```python
from build123d import *

# Parameters (mm, degrees)
SKETCH1_R                       = 3
SKETCH1_R_2                     = 6
BOSS_EXTRUDE1_DEPTH             = 6
M4X0_7_TAPPED_HOLE1_D           = 3.3
CHAMFER1_SIZE                   = 3
CHAMFER2_SIZE                   = 1
BOSS_EXTRUDE2_DEPTH             = 4.25
M4X0_7_START                    = -20.526744186
M4X0_7_TAPPED_HOLE3_OUTLINE_R   = 1.65
M4X0_7_TAPPED_HOLE3_DEPTH       = 1.123131525
M4X0_7_START_2                  = -19.403612661
M4X0_7_TAPPED_HOLE3_2_OUTLINE_R = 1.65
M4X0_7_TAPPED_HOLE3_2_DEPTH     = 0.494491736
M4X0_7_START_3                  = -6.0000001
M4X0_7_TAPPED_HOLE3_3_DEPTH     = 6.0000002
M4X0_7_START_4                  = -6.7750001
M4X0_7_TAPPED_HOLE3_4_DEPTH     = 0.775
SKETCH14_R                      = 3
CUT_EXTRUDE1_DEPTH              = 87.67199356


with BuildPart() as part:
    # Sketch1 → Boss-Extrude1 (new body)
    with BuildSketch(Plane.XY):
        with BuildLine():
            Line((62.473255814, 56.275636954), (55.545052584, 60.275636954))
            Line((55.545052584, 60.275636954), (24.782656891, 6.993604651))
            ThreePointArc((24.782656891, 6.993604651), (21.122402853, 3.333350613), (16.122402853, 1.993604651))
            Line((16.122402853, 1.993604651), (-20.526744186, 1.993604651))
            Line((-20.526744186, 1.993604651), (-20.526744186, -13.006395349))
            Line((-20.526744186, -13.006395349), (22.473255814, -13.006395349))
            Line((22.473255814, -13.006395349), (62.473255814, 56.275636954))
        make_face()
        with Locations((-16.403612561, -5.506395349)):
            Circle(SKETCH1_R, mode=Mode.SUBTRACT)
        with Locations((17.535345593, -5.506395349)):
            Circle(SKETCH1_R_2, mode=Mode.SUBTRACT)
    extrude(amount=-BOSS_EXTRUDE1_DEPTH)

    # M4x0.7 Tapped Hole1 (through all)
    with Locations(Plane.XY):
        with Locations((36.509154199, 19.304493784)):
            Hole(M4X0_7_TAPPED_HOLE1_D / 2)

    # Chamfer1
    chamfer1_edges = [part.edges().sort_by_distance(p)[0] for p in [
        (-20.526744186, -13.006395349, -3),
    ]]
    chamfer(chamfer1_edges, length=CHAMFER1_SIZE)

    # Chamfer2
    chamfer2_edges = [part.edges().sort_by_distance(p)[0] for p in [
        (42.473255814, 21.634620803, -6),
        (55.545052584, 60.275636954, -3),
        (42.473255814, 21.634620803, 0),
    ]]
    chamfer(chamfer2_edges, length=CHAMFER2_SIZE)

    # Sketch6 → Boss-Extrude2 (add)
    with BuildSketch(Plane(origin=(0, 0, -6), x_dir=(-1, 0, 0), z_dir=(0, 0, -1))):
        Polygon((20.526744186, 1.993604651), (1.306644629, 1.993604651), (1.306644629, -13.006395349), (17.526744186, -13.006395349), (20.526744186, -10.006395349), align=None)
    extrude(amount=BOSS_EXTRUDE2_DEPTH)

    # M4x0.7 Tapped Hole3: read off the stored shape, not the designer's step
    # M4x0.7 Tapped Hole3 outline → M4x0.7 Tapped Hole3 (cut)
    with BuildSketch(Plane.YZ.offset(M4X0_7_START)):
        with Locations((-5.506395349, -5.125)):
            Circle(M4X0_7_TAPPED_HOLE3_OUTLINE_R)
    extrude(amount=M4X0_7_TAPPED_HOLE3_DEPTH, mode=Mode.SUBTRACT)

    # M4x0.7 Tapped Hole3 2 outline → M4x0.7 Tapped Hole3 2 (cut)
    with BuildSketch(Plane.YZ.offset(M4X0_7_START_2)):
        with Locations((-5.506395349, -5.125)):
            Circle(M4X0_7_TAPPED_HOLE3_2_OUTLINE_R)
    extrude(amount=M4X0_7_TAPPED_HOLE3_2_DEPTH, mode=Mode.SUBTRACT)

    # M4x0.7 Tapped Hole3 3 outline → M4x0.7 Tapped Hole3 3 (cut)
    with BuildSketch(Plane.XY.offset(M4X0_7_START_3)):
        with BuildLine():
            ThreePointArc((-18.909118414, -3.856413403), (-18.986363136, -3.980158321), (-19.057501217, -4.107511865))
            ThreePointArc((-19.057501217, -4.107511865), (-19.403612561, -5.506395898), (-19.057500704, -6.905279805))
            ThreePointArc((-19.057500704, -6.905279805), (-18.98636247, -7.032633505), (-18.909117577, -7.156378566))
            Line((-18.909117577, -7.156378566), (-18.909118414, -3.856413403))
        make_face()
    extrude(amount=M4X0_7_TAPPED_HOLE3_3_DEPTH, mode=Mode.SUBTRACT)

    # M4x0.7 Tapped Hole3 4 outline → M4x0.7 Tapped Hole3 4 (add)
    with BuildSketch(Plane.XY.offset(M4X0_7_START_4)):
        with BuildLine():
            ThreePointArc((-18.909118414, -3.856413403), (-18.986363136, -3.980158321), (-19.057501217, -4.107511865))
            ThreePointArc((-19.057501217, -4.107511865), (-19.403612561, -5.506395898), (-19.057500704, -6.905279805))
            ThreePointArc((-19.057500704, -6.905279805), (-18.98636247, -7.032633505), (-18.909117577, -7.156378566))
            Line((-18.909117577, -7.156378566), (-18.909118414, -3.856413403))
        make_face()
    extrude(amount=M4X0_7_TAPPED_HOLE3_4_DEPTH)

    # Sketch14 → Cut-Extrude1 (cut, through all)
    with BuildSketch(Plane.XY.offset(-6)):
        with Locations((-16.403612561, -5.506395349)):
            Circle(SKETCH14_R)
    extrude(amount=-CUT_EXTRUDE1_DEPTH, mode=Mode.SUBTRACT)


solid = part.part
```
Geometry: final body of the model. Coordinates: model frame, mm. A direction names the side the tool comes from. Round coordinates to 2 decimals unless told otherwise and drop trailing zeros. Order: outer loops, then holes, each group sorted by start corner. A loop starts at its lowest first (then second) coordinate and runs counter-clockwise, first axis right, second up. Notation, with made-up numbers: (3, -27) -> (42, -27) arc R12 ccw to (42, -15) -> close; hole circle Ø2 at (10, -30.5). An arc over 180 degrees is marked (long way). Use CSV: the item, a comma, the result in double quotes. Start each with the question number.
1) Material intervals for line 1 along X through (y, z) = (-3.5, -0.5); line 2 along Y through (x, z) = (-0.5, -3); line 3 along Z through (x, y) = (29.5, 8.5), sorted ascending. Write a range as from..to.
2) Section A-A (z = -8). Return the cut outline in (x, y), and give its area (3 significant figures).
3) Section C-C (y = 46.5). Return the cut outline in (x, z), and give its area (3 significant figures).
4) Draft query along X for faces 6 (the face through (-19.006, -11.527, -5.053)), 7 (the face through (35.622, 20.696, -3.042)), 8 (the face through (59.485, 58.001, -2.958)). Return one class per face: +X half, -X half, draft (parallel to the pull), parting line (faces both ways), or undercut.
5) First-contact query: pin 1 Ø4.5 at (y, z) = (-4.5, -8.5) entering from +X; pin 2 Ø4.5 at (x, y) = (36.51, 19.3) entering from +Z; pin 3 Ø2.5 at (y, z) = (-5.51, -5.12) entering from -X; pin 4 Ø4 at (y, z) = (1, -1.5) entering from +X. Flat tips, straight axial feed; report the tip coordinate or a pass-through.
6) Section B-B (x = 0). Return the cut outline in (y, z).
7) Set-up query: faces 1 (the face through (41.608, 21.15, -5.507)), 2 (the face through (-7, 1.994, -4)), 3 (the face through (-19.9, -4, -5.8)), 4 (the face through (30, 15, -6)), 5 (the face through (-13.54, -4.61, -5.05)). Return all of +Z, -Z, +X, -X, +Y, -Y with unobstructed straight access to the full face (end or side cutting, diameter ignored); none if empty.
8) Section D-D (x = -11.5). Return the cut outline in (y, z), and give its area (3 significant figures).
Returned:
1,line 1,"x = -20.53..-18.63, -14.17..11.88, 23.19..27.38"
1,line 2,"y = -13.01..1.99"
1,line 3,"z = -6..0"
2,outline,"(-20.53, -10.01) -> (-17.53, -13.01) -> (-1.31, -13.01) -> (-1.31, 1.99) -> (-20.53, 1.99) -> close; hole circle Ø6 at (-16.4, -5.51)"
2,area,"256 mm²"
3,outline,"(47.59, -6) -> (55.67, -6) -> (56.83, -5) -> (56.83, -1) -> (55.67, 0) -> (47.59, 0) -> close"
3,area,"54.3 mm²"
4,face 6,"-X half"
4,face 7,"undercut"
4,face 8,"+X half"
5,pin 1,"stops at x = -1.31"
5,pin 2,"stops at z = 0"
5,pin 3,"stops at x = -13.68"
5,pin 4,"stops at x = 31.71"
6,outline,"(-13.01, -6) -> (1.99, -6) -> (1.99, 0) -> (-13.01, 0) -> close"
7,face 1,"-Z, +X, -Y"
7,face 2,"+Z, -Z, -X, +Y"
7,face 3,"-X"
7,face 4,"-Z, +X, +Y, -Y"
7,face 5,"+Z, -Z"
8,outline,"(-13.01, -10.25) -> (1.99, -10.25) -> (1.99, 0) -> (-13.01, 0) -> close"
8,area,"154 mm²"
